from build123d import *

# Parameters (mm, degrees)
F0_W      = 43.7
F0_H      = 42.4
F1_DEPTH  = 20
F2_W      = 41.7
F2_H      = 40.4
F3_DEPTH  = 19
F4_R      = 1.5
F5_DEPTH  = 1
F6_R      = 4.5
F7_DEPTH  = 1
F8_W      = 15
F8_H      = 12
F9_DEPTH  = 1
F10_W     = 20
F10_H     = 14.5
F11_DEPTH = 1
F12_W     = 3.5
F12_H     = 2
F13_DEPTH = 1


with BuildPart() as f1:
    # F0 (on Top) → F1 (new body)
    with BuildSketch(Plane.XY):
        with Locations((-21.85, 26.01227)):
            Rectangle(F0_W, F0_H)
    extrude(amount=F1_DEPTH)

    # F2 (on face) → F3 (cut)
    with BuildSketch(Plane.XY.offset(20)):
        with Locations((-21.85, 26.01227)):
            Rectangle(F2_W, F2_H)
    extrude(amount=-F3_DEPTH, mode=Mode.SUBTRACT)

    # F4 (on face) → F5 (cut)
    with BuildSketch(Plane.XY.offset(1)):
        with Locations((-5, 42.21227)):
            Circle(F4_R)
        with Locations((-36.4, 9.81227)):
            Circle(F4_R)
    extrude(amount=-F5_DEPTH, mode=Mode.SUBTRACT)

    # F6 (on face) → F7 (cut)
    with BuildSketch(Plane.XY.offset(1)):
        with Locations((-21.1, 36.21227)):
            Circle(F6_R)
    extrude(amount=-F7_DEPTH, mode=Mode.SUBTRACT)

    # F8 (on face) → F9 (cut)
    with BuildSketch(Plane(origin=(-43.7, 0, 0), x_dir=(0, -1, 0), z_dir=(-1, 0, 0))):
        with Locations((-22.31227, 11.5)):
            Rectangle(F8_W, F8_H)
    extrude(amount=-F9_DEPTH, mode=Mode.SUBTRACT)

    # F10 (on face) → F11 (cut)
    with BuildSketch(Plane.XZ.offset(-4.81227)):
        with Locations((-12, 12.75)):
            Rectangle(F10_W, F10_H)
    extrude(amount=-F11_DEPTH, mode=Mode.SUBTRACT)

    # F12 (on face) → F13 (cut)
    with BuildSketch(Plane(origin=(0, 0, 0), x_dir=(1, 0, 0), z_dir=(0, 0, -1))):
        with Locations((-33.95, -13.81227)):
            Rectangle(F12_W, F12_H)
    extrude(amount=-F13_DEPTH, mode=Mode.SUBTRACT)


solid = f1.part
The model under review builds one solid part; all positions refer to its coordinate system, in mm. A direction names the side the tool comes from. Round coordinates to 2 decimals unless told otherwise and drop trailing zeros. Order: outer loops, then holes, each group sorted by start corner. A loop starts at its lowest first (then second) coordinate and runs counter-clockwise, first axis right, second up. Notation, with made-up numbers: (-32, 87) -> (6, 87) arc R34 cw to (6, 122) -> close; hole circle Ø2 at (-14.75, 47). An arc over 180 degrees is marked (long way). Write item = value, one per line. Start each with the question number.
Item 1: Consider section A-A on y = 13.5. Write out the cut boundary in (x, z), plus the area to 3 significant figures.
Item 2: For faces 4 (the face through (-32.2, 13.8, 0.5)), 5 (the face through (-27, 5.812, 9)), 6 (the face through (-22, 5, 13)), 7 (the face through (0, 26, 10)), 8 (the face through (-43, 22, 5.5)), list the 3-axis set-ups (+Z, -Z, +X, -X, +Y, -Y) from which the entire face can be reached by the end or side of a thin tool; tool diameter is ignored.
Item 3: Mouldability with a two-part tool opening along Y and no side actions: class faces 1 (the face through (-22, 47.212, 10)), 2 (the face through (-22, 46.212, 11)), 3 (the face through (-24, 47, 20)) as released by +Y, released by -Y, zero draft, split by the parting line, or undercut.
Item 4: Consider section C-C on z = 3.75. Write out the cut boundary in (x, y).
Item 5: Clearance check with flat-ended pins moving along their axes: pin 1 Ø1 at (x, y) = (-26.5, 33) entering from +Z; pin 2 Ø3 at (x, z) = (-6, 14) entering from -Y. State where each tip first meets the part, or that it passes through.
Item 6: Consider section B-B on x = -36.4. Write out the cut boundary in (y, z), plus the area to 3 significant figures.
Item 7: For line 1 along Y through (x, z) = (-36.4, 0.65); line 2 along X through (y, z) = (17, 2.5); line 3 along Y through (x, z) = (-40.5, 15), list the stretches that pass through material, from the lowest coordinate up.
Item 8: Consider section D-D on x = -12. Write out the cut boundary in (y, z), plus the area to 3 significant figures.
Conclusion:
q1.outline = (-43.7, 0) -> (-35.7, 0) -> (-35.7, 1) -> (-42.7, 1) -> (-42.7, 20) -> (-43.7, 20) -> close; (-32.2, 0) -> (0, 0) -> (0, 20) -> (-1, 20) -> (-1, 1) -> (-32.2, 1) -> close
q1.area = 78.2 mm2
q2.face_4 = +Z, -Z
q2.face_5 = +Z
q2.face_6 = +Z, -Y
q2.face_7 = +Z, -Z, +X, +Y, -Y
q2.face_8 = -X
q3.face_1 = released by +Y
q3.face_2 = undercut
q3.face_3 = zero draft
q4.outline = (-43.7, 4.81) -> (0, 4.81) -> (0, 47.21) -> (-43.7, 47.21) -> close; hole (-42.7, 5.81) -> (-1, 5.81) -> (-1, 46.21) -> (-42.7, 46.21) -> close
q5.pin_1 = 1
q5.pin_2 = 46.21
q6.outline = (4.81, 0) -> (8.31, 0) -> (8.31, 1) -> (5.81, 1) -> (5.81, 20) -> (4.81, 20) -> close; (11.31, 0) -> (47.21, 0) -> (47.21, 20) -> (46.21, 20) -> (46.21, 1) -> (11.31, 1) -> close
q6.area = 77.4 mm2
q7.line_1 = 4.81 to 8.31, 11.31 to 47.21
q7.line_2 = -43.7 to -42.7, -1 to 0
q7.line_3 = 4.81 to 5.81, 46.21 to 47.21
q8.outline = (4.81, 0) -> (47.21, 0) -> (47.21, 20) -> (46.21, 20) -> (46.21, 1) -> (5.81, 1) -> (5.81, 5.5) -> (4.81, 5.5) -> close
q8.area = 65.9 mm2
